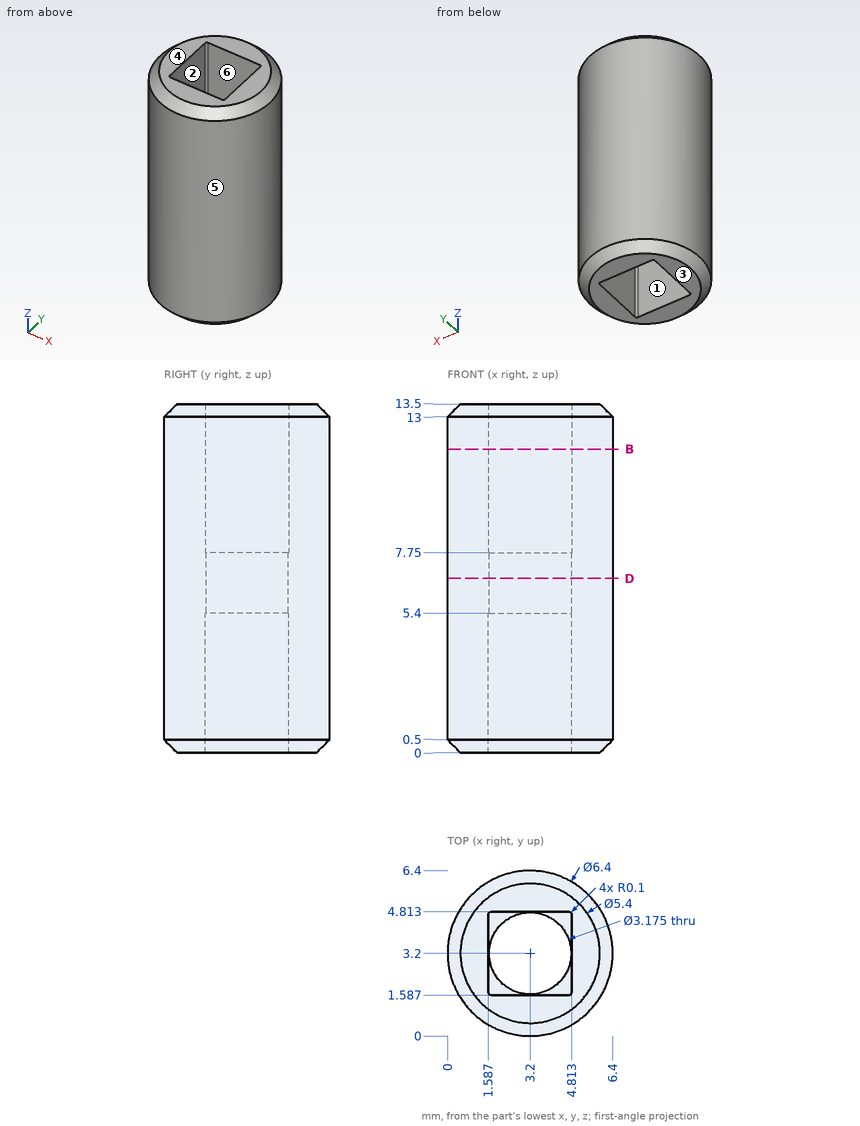
Input: dimensioned drawing with shaded views. Units: mm. Origin: part minimum x, y, z. A direction names the side the tool comes from. Give positions to 0.01 mm unless a question says otherwise; leave off trailing zeros. Loops run counter-clockwise (first coordinate to the right, second up) from the corner with the lowest first, then second, coordinate; pieces in that order, holes last. Notation, with made-up numbers: (57, 57.5) -> (74, 57.5) arc R12 cw to (74, 61.5) -> close; hole circle Ø10 at (64, -27.5). An arc over 180 degrees is marked (long way). Return JSON: item names as keys, results as strings.
Item 1: Line query: line 1 (Y direction, x = 3.2, z = 7.3); line 2 (X direction, y = 4, z = 11.5); line 3 (X direction, y = 2, z = 1.75). Output: solid intervals per line, ascending.
Filled in:
{"line 1": "0 to 1.61, 4.79 to 6.4", "line 2": "0.1 to 1.59, 4.81 to 6.3", "line 3": "0.23 to 1.59, 4.81 to 6.17"}
Item 2: Access query for the marked faces 1, 2 and 3. Directions: +Z, -Z, +X, -X, +Y, -Y. A direction counts if a zero-diameter tool reaches every point of the face in a straight line with its end or side. Return the directions, or none.
Filled in:
{"face 1": "-Z", "face 2": "+Z", "face 3": "-Z, +X, -X, +Y, -Y"}
Item 3: Mould query, pull axis Y, two halves, no side actions, for the marked faces 4, 5 and 6. Classes: released by +Y, released by -Y, zero draft, split by the parting line, or undercut.
Filled in:
{"face 4": "zero draft", "face 5": "split by the parting line", "face 6": "undercut"}
Item 4: Pin query (flat end, axial travel): P1, Ø0.9, axis at y = 2.5, z = 10.5, coming from the +X side; P2, Ø3, axis at y = 5.5, z = 6, coming from the -X side; P3, Ø1.5, axis at x = 5, z = 7.5, coming from the +Y side; P4, Ø1.6, axis at x = 3.5, y = 3, coming from the +Z side. Return the tip coordinate at first contact, or that it passes through.
Filled in:
{"P1": "x = 6.39", "P2": "x = 0.1", "P3": "y = 6.22", "P4": "through"}
Item 5: Section B-B, the plane z = 11.75. Output: boundary loops of the cut face in (x, y).
Filled in:
{"outline": "circle Ø6.4 at (3.2, 3.2); hole (1.59, 1.69) arc R0.1 ccw to (1.69, 1.59) -> (4.71, 1.59) arc R0.1 ccw to (4.81, 1.69) -> (4.81, 4.71) arc R0.1 ccw to (4.71, 4.81) -> (1.69, 4.81) arc R0.1 ccw to (1.59, 4.71) -> close"}
Item 6: Section D-D, the plane z = 6.75. Output: boundary loops of the cut face in (x, y) (1 decimal).
Filled in:
{"outline": "circle Ø6.4 at (3.2, 3.2); hole circle Ø3.2 at (3.2, 3.2)"}
